Model file for the job. Use its own axes, mm. Face numbers are marked on the shaded views. A direction names the side the tool comes from. Give positions to 0.01 mm unless a question says otherwise; leave off trailing zeros. Loops run counter-clockwise (first coordinate to the right, second up) from the corner with the lowest first, then second, coordinate; pieces in that order, holes last. Notation, with made-up numbers: M 19,-38.75 L 50,-38.75 A19 cw 50,-26.75 Z; hole C 29.5,54.5 d6. An arc over 180 degrees is marked long. Answer in a Markdown table with one row per item.
```python
from build123d import *

# Parameters (mm, degrees)
SKETCH1_W                  = 320
SKETCH1_H                  = 38.1
SKETCH1_R                  = 2.5
BASE_FLANGE1_DEPTH         = 6.4
CHAMFER2_SIZE              = 5
SKETCH32_R                 = 5
CUT_EXTRUDE2_DEPTH         = 3
SKETCHED_START             = 4.650863044
SKETCHED_BEND1_OUTLINE_W   = 38.1
SKETCHED_BEND1_OUTLINE_H   = 6.4
SKETCHED_BEND1_DEPTH       = 155.349136956
SKETCHED_START_2           = -2.499136956
SKETCHED_BEND1_2_OUTLINE_R = 2.5
SKETCHED_BEND1_2_DEPTH     = 7.15
SKETCHED_START_3           = -20
SKETCHED_BEND1_3_DEPTH     = 40


with BuildPart() as part:
    # Base-Flange1: sheet metal written as solids
    # Sketch1 → Base-Flange1 (new body)
    with BuildSketch(Plane.XY):
        Rectangle(SKETCH1_W, SKETCH1_H)
        with Locations((-145, 10)):
            Circle(SKETCH1_R, mode=Mode.SUBTRACT)
        with Locations((-125, 10)):
            Circle(SKETCH1_R, mode=Mode.SUBTRACT)
        with Locations((-105, 10)):
            Circle(SKETCH1_R, mode=Mode.SUBTRACT)
        with Locations((-85, 10)):
            Circle(SKETCH1_R, mode=Mode.SUBTRACT)
        with Locations((-65, 10)):
            Circle(SKETCH1_R, mode=Mode.SUBTRACT)
        with Locations((-45, 10)):
            Circle(SKETCH1_R, mode=Mode.SUBTRACT)
        with Locations(Location((-145, -10, 0), (0, 0, 180))):
            Circle(SKETCH1_R, mode=Mode.SUBTRACT)
        with Locations(Location((-125, -10, 0), (0, 0, 180))):
            Circle(SKETCH1_R, mode=Mode.SUBTRACT)
        with Locations(Location((-105, -10, 0), (0, 0, 180))):
            Circle(SKETCH1_R, mode=Mode.SUBTRACT)
        with Locations(Location((-85, -10, 0), (0, 0, 180))):
            Circle(SKETCH1_R, mode=Mode.SUBTRACT)
        with Locations(Location((-65, -10, 0), (0, 0, 180))):
            Circle(SKETCH1_R, mode=Mode.SUBTRACT)
        with Locations(Location((-45, -10, 0), (0, 0, 180))):
            Circle(SKETCH1_R, mode=Mode.SUBTRACT)
        with Locations((140, 10)):
            Circle(SKETCH1_R, mode=Mode.SUBTRACT)
        with Locations((120, 10)):
            Circle(SKETCH1_R, mode=Mode.SUBTRACT)
        with Locations((120, -10)):
            Circle(SKETCH1_R, mode=Mode.SUBTRACT)
        with Locations((140, -10)):
            Circle(SKETCH1_R, mode=Mode.SUBTRACT)
    extrude(amount=-BASE_FLANGE1_DEPTH)

    # Chamfer2
    chamfer2_edges = [part.edges().sort_by_distance(p)[0] for p in [
        (-160, 19.05, -3.2),
        (160, 19.05, -3.2),
        (160, -19.05, -3.2),
        (-160, -19.05, -3.2),
    ]]
    chamfer(chamfer2_edges, length=CHAMFER2_SIZE)

    # Sketch32 → Cut-Extrude2 (cut)
    with BuildSketch(Plane.XY):
        with Locations((-145, 10)):
            Circle(SKETCH32_R)
        with Locations((-125, 10)):
            Circle(SKETCH32_R)
        with Locations((-105, 10)):
            Circle(SKETCH32_R)
        with Locations((-85, 10)):
            Circle(SKETCH32_R)
        with Locations((-65, 10)):
            Circle(SKETCH32_R)
        with Locations((-45, 10)):
            Circle(SKETCH32_R)
        with Locations(Location((-45, -10, 0), (0, 0, 180))):
            Circle(SKETCH32_R)
        with Locations(Location((-65, -10, 0), (0, 0, 180))):
            Circle(SKETCH32_R)
        with Locations(Location((-85, -10, 0), (0, 0, 180))):
            Circle(SKETCH32_R)
        with Locations(Location((-105, -10, 0), (0, 0, 180))):
            Circle(SKETCH32_R)
        with Locations(Location((-125, -10, 0), (0, 0, 180))):
            Circle(SKETCH32_R)
        with Locations(Location((-145, -10, 0), (0, 0, 180))):
            Circle(SKETCH32_R)
    extrude(amount=-CUT_EXTRUDE2_DEPTH, mode=Mode.SUBTRACT)

    # Sketched Bend1: read off the stored shape, not the designer's step
    # Sketched Bend1 outline → Sketched Bend1 (cut)
    with BuildSketch(Plane.YZ.offset(SKETCHED_START)):
        with Locations((0, -3.2)):
            Rectangle(SKETCHED_BEND1_OUTLINE_W, SKETCHED_BEND1_OUTLINE_H)
    extrude(amount=SKETCHED_BEND1_DEPTH, mode=Mode.SUBTRACT)

    # Sketched Bend1 2 outline → Sketched Bend1 2 (add)
    with BuildSketch(Plane.YZ.offset(SKETCHED_START_2)):
        Polygon((-19.05, 0), (19.05, 0), (19.05, 153.250863044), (14.05, 158.250863044), (-14.05, 158.250863044), (-19.05, 153.250863044), align=None)
        with Locations((-10, 118.250863044)):
            Circle(SKETCHED_BEND1_2_OUTLINE_R, mode=Mode.SUBTRACT)
        with Locations((-10, 138.250863044)):
            Circle(SKETCHED_BEND1_2_OUTLINE_R, mode=Mode.SUBTRACT)
        with Locations((10, 118.250863044)):
            Circle(SKETCHED_BEND1_2_OUTLINE_R, mode=Mode.SUBTRACT)
        with Locations((10, 138.250863044)):
            Circle(SKETCHED_BEND1_2_OUTLINE_R, mode=Mode.SUBTRACT)
    extrude(amount=SKETCHED_BEND1_2_DEPTH)

    # Sketched Bend1 3 outline → Sketched Bend1 3 (cut)
    with BuildSketch(Plane(origin=(0, 0, 0), x_dir=(1, 0, 0), z_dir=(0, 1, 0)).offset(SKETCHED_START_3)):
        with BuildLine():
            Line((4.650863044, 6.4), (-2.499136956, 6.4))
            ThreePointArc((-2.499136956, 6.4), (2.55667653, 4.305813485), (4.650863044, -0.75))
            Line((4.650863044, -0.75), (4.650863044, 6.4))
        make_face()
        with BuildLine():
            Line((-2.499136956, -158.250863044), (-1.749136956, -158.250863044))
            Line((-1.749136956, -158.250863044), (-1.749136956, -0.75))
            ThreePointArc((-1.749136956, -0.75), (-1.96880687, -0.219669914), (-2.499136956, 0))
            Line((-2.499136956, 0), (-2.499136956, -158.250863044))
        make_face()
    extrude(amount=SKETCHED_BEND1_3_DEPTH, mode=Mode.SUBTRACT)


solid = part.part
```
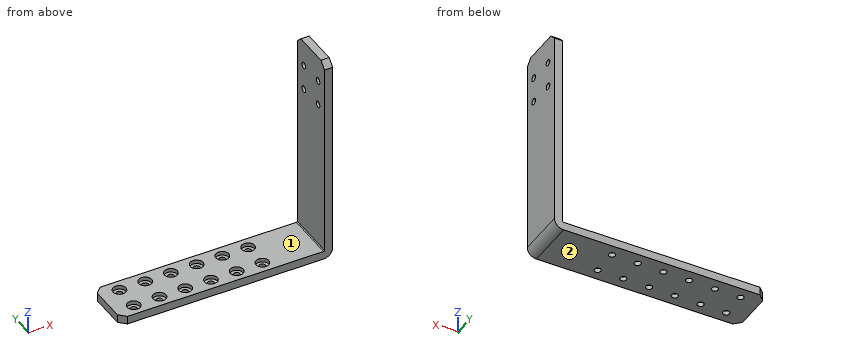
Q1. Saw through at A-A (x = -125). Give the cut face in (y, z), and give its area (3 significant figures).
Reported:
| item | result |
|---|---|
| outline | M -19.05,-6.4 L -12.5,-6.4 L -12.5,-3 L -15,-3 L -15,0 L -19.05,0 Z; M -7.5,-6.4 L 7.5,-6.4 L 7.5,-3 L 5,-3 L 5,0 L -5,0 L -5,-3 L -7.5,-3 Z; M 12.5,-6.4 L 19.05,-6.4 L 19.05,0 L 15,0 L 15,-3 L 12.5,-3 Z |
| area | 150 mm² |
Q2. Saw through at B-B (y = 10). Give the number of separate pieces and of enclosed holes in the cut face, and give its area (3 significant figures).
Reported:
| item | result |
|---|---|
| separate pieces | 9 |
| enclosed holes | 0 |
| area | 1,710 mm² |
Q3. Probe probe 1 along Y at (x, z) = (-105, -1); probe 2 along X at (y, z) = (-12, 79.5); probe 3 along Z at (x, y) = (-109, 8). List the from-to ranges inside material, lowest first.
Reported:
| item | result |
|---|---|
| probe 1 | -19.05 to -15, -5 to 5, 15 to 19.05 |
| probe 2 | -1.75 to 4.65 |
| probe 3 | -6.4 to -3 |
Q4. Saw through at C-C (z = 109). Give the cut face in (x, y).
Reported:
| item | result |
|---|---|
| outline | M -1.75,-19.05 L 4.65,-19.05 L 4.65,19.05 L -1.75,19.05 Z |
Q5. Drop flat-ended pins along their axis: pin 1 (6 mm diameter, centred on x = -125, y = -10, fed in from +Z); pin 2 (13 mm diameter, centred on x = -85, y = -10, fed in from +Z); pin 3 (4.5 mm diameter, centred on y = 10, z = 138.25, fed in from +X); pin 4 (6 mm diameter, centred on y = -10, z = 138.25, fed in from -X). Give the stop position or say it passes through.
Reported:
| item | result |
|---|---|
| pin 1 | z = -3 |
| pin 2 | z = 0 |
| pin 3 | through |
| pin 4 | x = -1.75 |
Q6. 3-axis set-ups, long thin cutter, end or side, ignore diameter. For the marked faces 1 and 2: which of +Z, -Z, +X, -X, +Y, -Y reach the whole face in a straight line?
Reported:
| item | result |
|---|---|
| face 1 | +Z, -X, +Y, -Y |
| face 2 | -Z, +X, -X, +Y, -Y |
